For this review, take the finished solid that the model builds, in its own axes (mm). Coordinates: 2 decimals unless noted, no trailing zeros. Loops run counter-clockwise (first coordinate to the right, second up) from the corner with the lowest first, then second, coordinate; pieces in that order, holes last. Notation, with made-up numbers: (-26, 31) - (10, 31) arc R18 cw to (10, 54) - close; hole circle Ø5 at (15.25, 33.5). An arc over 180 degrees is marked (long way). Use one line per item in the form item = value. Start each with the question number.
1. Add section A-A on x = 46.5. Give the boundary of the cut face in (y, z), and give its area (3 significant figures).
2. Add section C-C on x = 21.75. Give the boundary of the cut face in (y, z).
3. To check wall thickness, follow probe 1 along Y at (x, z) = (2.75, 1.85); probe 2 along X at (y, z) = (34, 1.45); probe 3 along Y at (x, z) = (7, 2). State the ranges of each line that lie inside material, in increasing order.
4. For pin 1 Ø1.2 at (x, z) = (24, 1) entering from -Y; pin 2 Ø0.8 at (x, z) = (29.5, 1.5) entering from +Y; pin 3 Ø1 at (x, z) = (26, 2) entering from -Y, all flat-tipped, find the tip position at first contact; note any pin that passes through.
5. Add section B-B on y = 5. Give the boundary of the cut face in (x, z), and give its area (3 significant figures).
6. Add section D-D on z = 0.4. Count the separate pieces of the cut face and the enclosed holes in it, and give its area (3 significant figures).
```python
from build123d import *

# Parameters (mm, degrees)
F0_R     = 1.6
F1_DEPTH = 2.5


with BuildPart() as f1:
    # F0 (on Top) → F1 (new body)
    with BuildSketch(Plane.XY):
        with BuildLine():
            Line((0, 17.25), (0, 0))
            Line((0, 0), (5.5, 0))
            Line((5.5, 0), (5.5, 10.75))
            Line((5.5, 10.75), (26.75, 10.75))
            Line((26.75, 10.75), (26.75, 32))
            Line((26.75, 32), (12.25, 32))
            Line((12.25, 32), (12.25, 23.25))
            ThreePointArc((12.25, 23.25), (11.37132, 21.12868), (9.25, 20.25))
            Line((9.25, 20.25), (3, 20.25))
            ThreePointArc((3, 20.25), (0.87868, 19.37132), (0, 17.25))
        make_face()
        with Locations((2.75, 5)):
            Circle(F0_R, mode=Mode.SUBTRACT)
        with BuildLine():
            Line((5.5, 0), (0, 0))
            Line((0, 0), (0, -17.25))
            ThreePointArc((0, -17.25), (0.87868, -19.37132), (3, -20.25))
            Line((3, -20.25), (9.25, -20.25))
            ThreePointArc((9.25, -20.25), (11.37132, -21.12868), (12.25, -23.25))
            Line((12.25, -23.25), (12.25, -32))
            Line((12.25, -32), (26.75, -32))
            Line((26.75, -32), (26.75, -10.75))
            Line((26.75, -10.75), (5.5, -10.75))
            Line((5.5, -10.75), (5.5, 0))
        make_face()
        with Locations((2.75, -5)):
            Circle(F0_R, mode=Mode.SUBTRACT)
        with BuildLine():
            Line((48, 10.75), (48, 0))
            Line((48, 0), (53.5, 0))
            Line((53.5, 0), (53.5, 17.25))
            ThreePointArc((53.5, 17.25), (52.62132, 19.37132), (50.5, 20.25))
            Line((50.5, 20.25), (44.25, 20.25))
            ThreePointArc((44.25, 20.25), (42.12868, 21.12868), (41.25, 23.25))
            Line((41.25, 23.25), (41.25, 32))
            Line((41.25, 32), (26.75, 32))
            Line((26.75, 32), (26.75, 10.75))
            Line((26.75, 10.75), (48, 10.75))
        make_face()
        with Locations((50.75, 5)):
            Circle(F0_R, mode=Mode.SUBTRACT)
        with BuildLine():
            Line((53.5, 0), (48, 0))
            Line((48, 0), (48, -10.75))
            Line((48, -10.75), (26.75, -10.75))
            Line((26.75, -10.75), (26.75, -32))
            Line((26.75, -32), (41.25, -32))
            Line((41.25, -32), (41.25, -23.25))
            ThreePointArc((41.25, -23.25), (42.12868, -21.12868), (44.25, -20.25))
            Line((44.25, -20.25), (50.5, -20.25))
            ThreePointArc((50.5, -20.25), (52.62132, -19.37132), (53.5, -17.25))
            Line((53.5, -17.25), (53.5, 0))
        make_face()
        with Locations((50.75, -5)):
            Circle(F0_R, mode=Mode.SUBTRACT)
        with BuildLine():
            Line((41.25, -32), (26.75, -32))
            Line((26.75, -32), (26.75, -39.4))
            ThreePointArc((26.75, -39.4), (27.704594, -39.795406), (28.1, -40.75))
            ThreePointArc((28.1, -40.75), (27.704594, -41.704594), (26.75, -42.1))
            Line((26.75, -42.1), (26.75, -46.5))
            ThreePointArc((26.75, -46.5), (37.003048, -42.253048), (41.25, -32))
        make_face()
        with Locations((31.75, -33.75)):
            Circle(F0_R, mode=Mode.SUBTRACT)
        with BuildLine():
            Line((26.75, -39.4), (26.75, -32))
            Line((26.75, -32), (12.25, -32))
            ThreePointArc((12.25, -32), (16.496952, -42.253048), (26.75, -46.5))
            Line((26.75, -46.5), (26.75, -42.1))
            ThreePointArc((26.75, -42.1), (25.4, -40.75), (26.75, -39.4))
        make_face()
        with Locations((21.75, -33.75)):
            Circle(F0_R, mode=Mode.SUBTRACT)
        with BuildLine():
            Line((12.25, 32), (26.75, 32))
            Line((26.75, 32), (26.75, 39.4))
            ThreePointArc((26.75, 39.4), (25.4, 40.75), (26.75, 42.1))
            Line((26.75, 42.1), (26.75, 46.5))
            ThreePointArc((26.75, 46.5), (16.496952, 42.253048), (12.25, 32))
        make_face()
        with Locations((21.75, 33.75)):
            Circle(F0_R, mode=Mode.SUBTRACT)
        with BuildLine():
            Line((26.75, 39.4), (26.75, 32))
            Line((26.75, 32), (41.25, 32))
            ThreePointArc((41.25, 32), (37.003048, 42.253048), (26.75, 46.5))
            Line((26.75, 46.5), (26.75, 42.1))
            ThreePointArc((26.75, 42.1), (27.704594, 41.704594), (28.1, 40.75))
            ThreePointArc((28.1, 40.75), (27.704594, 39.795406), (26.75, 39.4))
        make_face()
        with Locations((31.75, 33.75)):
            Circle(F0_R, mode=Mode.SUBTRACT)
    extrude(amount=F1_DEPTH)


solid = f1.part
```
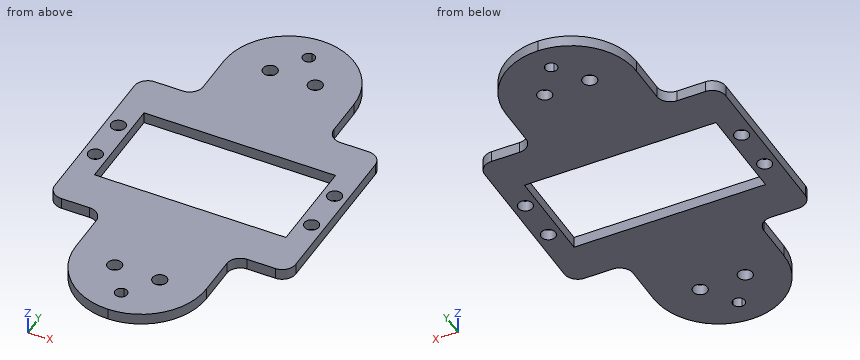
Conclusion:
q1.outline = (-20.25, 0) - (-10.75, 0) - (-10.75, 2.5) - (-20.25, 2.5) - close; (10.75, 0) - (20.25, 0) - (20.25, 2.5) - (10.75, 2.5) - close
q1.area = 47.5 mm^2
q2.outline = (-45.61, 0) - (-35.35, 0) - (-35.35, 2.5) - (-45.61, 2.5) - close; (-32.15, 0) - (-10.75, 0) - (-10.75, 2.5) - (-32.15, 2.5) - close; (10.75, 0) - (32.15, 0) - (32.15, 2.5) - (10.75, 2.5) - close; (35.35, 0) - (45.61, 0) - (45.61, 2.5) - (35.35, 2.5) - close
q3.probe_1 = -20.24 to -6.6, -3.4 to 3.4, 6.6 to 20.24
q3.probe_2 = 12.39 to 20.17, 23.33 to 30.17, 33.33 to 41.11
q3.probe_3 = -20.25 to -10.75, 10.75 to 20.25
q4.pin_1 = -46.34
q4.pin_2 = 46.31
q4.pin_3 = -46.5
q5.outline = (0, 0) - (1.15, 0) - (1.15, 2.5) - (0, 2.5) - close; (4.35, 0) - (5.5, 0) - (5.5, 2.5) - (4.35, 2.5) - close; (48, 0) - (49.15, 0) - (49.15, 2.5) - (48, 2.5) - close; (52.35, 0) - (53.5, 0) - (53.5, 2.5) - (52.35, 2.5) - close
q5.area = 11.5 mm^2
q6.separate_pieces = 1
q6.enclosed_holes = 11
q6.area = 2,520 mm^2
